Design review of the part shown in the three views and the two pictorial views. Dimensions are in mm from the part's minimum x, y and z. A direction names the side the tool comes from. Give positions to 0.01 mm unless a question says otherwise; leave off trailing zeros. Loops run counter-clockwise (first coordinate to the right, second up) from the corner with the lowest first, then second, coordinate; pieces in that order, holes last.
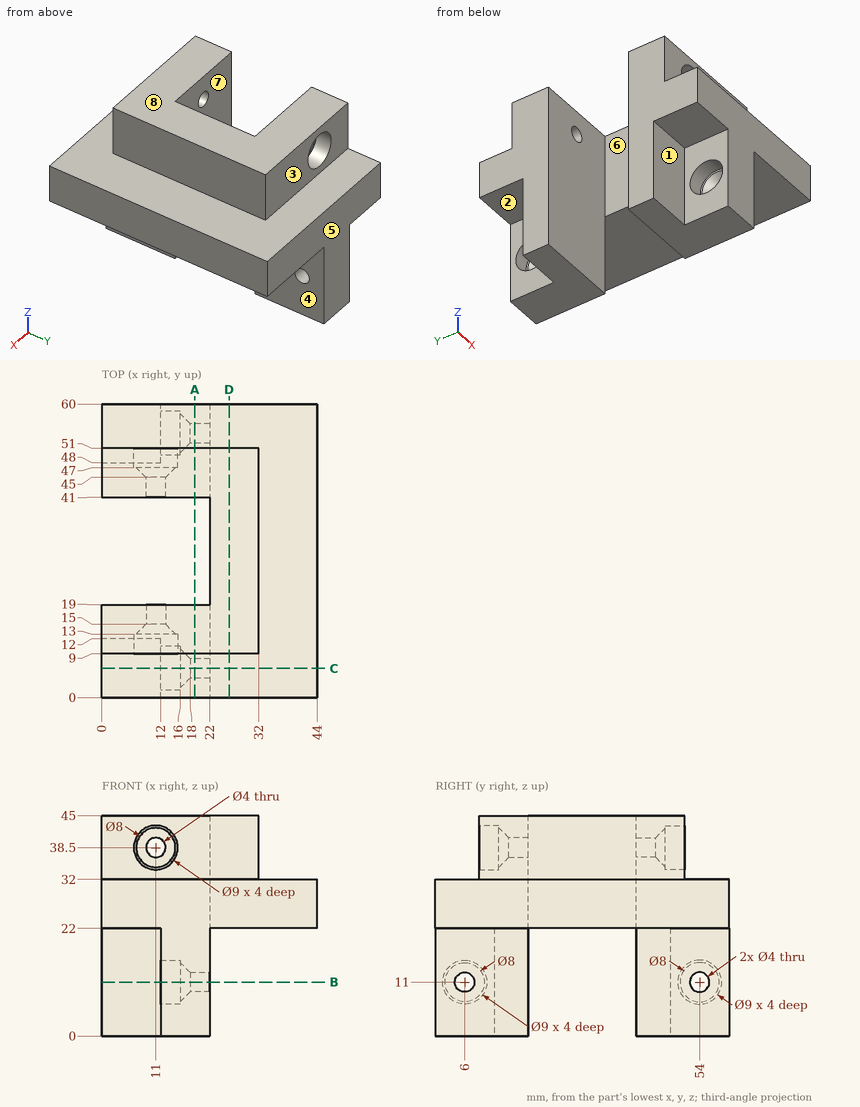
Q1. Mouldability with a two-part tool opening along Y and no side actions: class the marked faces 5, 6, 7 and 8 as +Y half, -Y half, draft (parallel to the pull), parting line (faces both ways), or undercut.
Answers:
face 5: +Y half
face 6: undercut
face 7: undercut
face 8: draft
Q2. Consider section D-D on x = 26. Give the boundary of the cut face in (y, z), plus the area to 3 significant figures.
Answers:
outline: (0, 22) - (60, 22) - (60, 32) - (51, 32) - (51, 45) - (9, 45) - (9, 32) - (0, 32) - close
area: 1,150 mm2
Q3. Consider section C-C on y = 6. Give the boundary of the cut face in (x, z), plus the area to 3 significant figures.
Answers:
outline: (0, 22) - (12, 22) - (12, 15.5) - (16, 15.5) - (16, 15) - (18, 13) - (22, 13) - (22, 22) - (44, 22) - (44, 32) - (0, 32) - close; (12, 0) - (22, 0) - (22, 9) - (18, 9) - (16, 7) - (16, 6.5) - (12, 6.5) - close
area: 596 mm2
Q4. Consider section B-B on z = 11. Count the separate pieces of the cut face and the enclosed holes in it, plus the area to 3 significant figures.
Answers:
separate pieces: 4
enclosed holes: 0
area: 420 mm2
Q5. For probe 1 along Y at (x, z) = (14.75, 11); probe 2 along Y at (x, z) = (10, 14); probe 3 along Y at (x, z) = (21, 22.5), list the stretches that pass through material, from the lowest coordinate up.
Answers:
probe 1: y = 0 to 1.5, 10.5 to 19, 41 to 49.5, 58.5 to 60
probe 2: y = 12 to 19, 41 to 48
probe 3: y = 0 to 19, 41 to 60
Q6. Machinability: for the marked faces 1, 2, 3 and 4, which of the approach directions +Z, -Z, +X, -X, +Y, -Y give a long, thin tool a straight path to every point of the face, cutting with its end or side? Answer none if there is none.
Answers:
face 1: -Z, -X, -Y
face 2: -Z, -X, +Y
face 3: +Z, +X, -X, +Y
face 4: -Z, +X, +Y, -Y
Q7. For pin 1 Ø11.5 at (y, z) = (54, 11) entering from -X; pin 2 Ø10 at (y, z) = (44.5, 38.5) entering from +X; pin 3 Ø3.5 at (x, y) = (3, 56.5) entering from -Z; pin 4 Ø3 at (x, z) = (11, 38.5) entering from +Y, all flat-tipped, find the tip position at first contact; note any pin that passes through.
Answers:
pin 1: stops at x = 12
pin 2: stops at x = 32
pin 3: stops at z = 22
pin 4: passes through
Q8. Consider section A-A on x = 19. Give the boundary of the cut face in (y, z).
Answers:
outline: (0, 0) - (19, 0) - (19, 45) - (9, 45) - (9, 32) - (0, 32) - close; (41, 0) - (60, 0) - (60, 32) - (51, 32) - (51, 45) - (41, 45) - close; hole circle Ø4 at (6, 11); hole circle Ø4 at (54, 11)
